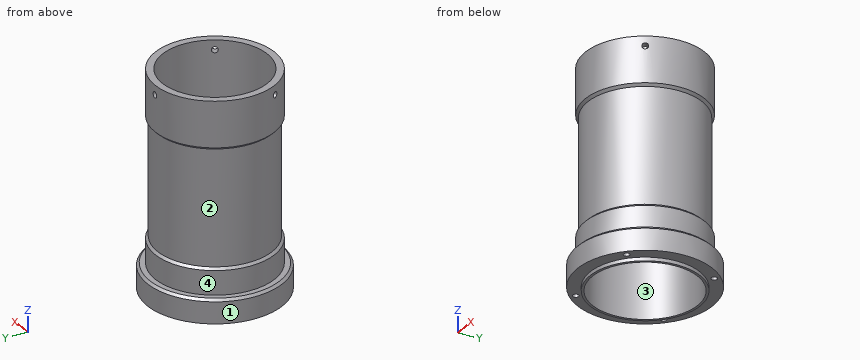
```python
from build123d import *

# Parameters (mm, degrees)
HOLE_WIZARD_M3_1_D       = 2.5
HOLE_WIZARD_M3_1_DEPTH   = 7
HOLE_WIZARD_M3_1_TIP     = 0.751075774
CHAMFER_2_SIZE           = 1
SKETCH_20_W              = 1.25
SKETCH_20_H              = 28.25
PATTERN_CIRCULAR_1_COUNT = 3


with BuildPart() as part:
    # 草图1 → 旋转1 (revolve)
    with BuildSketch(Plane(origin=(0, 0, 0), x_dir=(1, 0, 0), z_dir=(0, 1, 0))):
        Polygon((25, 0), (25, 19), (24, 19), (24, 69), (25, 69), (25, 79), (28.25, 79), (28.25, 89), (23, 89), (23, 90.5), (22, 90.5), (22, 0), align=None)
    revolve(axis=Axis((0, 0, 0), (0, 0, -1)))

    # M3 螺纹孔1
    with Locations(Plane(origin=(0, 0, -89), x_dir=(-1, 0, 0), z_dir=(0, 0, -1))):
        with Locations((-18.207999616, 18.207999616), (18.207999616, 18.207999616), (18.207999616, -18.207999616), (-18.207999616, -18.207999616)):
            Hole(HOLE_WIZARD_M3_1_D / 2, depth=HOLE_WIZARD_M3_1_DEPTH)
            with Locations((0, 0, -(HOLE_WIZARD_M3_1_DEPTH + HOLE_WIZARD_M3_1_TIP / 2))):  # 118° drill point
                Cone(0, HOLE_WIZARD_M3_1_D / 2, HOLE_WIZARD_M3_1_TIP, mode=Mode.SUBTRACT)

    # 倒角2
    chamfer_2_edges = [part.edges().sort_by_distance(p)[0] for p in [
        (-28.25, 0, -79),
        (-24, 0, -69),
        (-24, 0, -19),
    ]]
    chamfer(chamfer_2_edges, length=CHAMFER_2_SIZE - 0.0001)  # a hair under: the kernel refuses the full size

    # 草图20 → M3 螺纹孔2 (revolve, cut)
    with BuildSketch(Plane(origin=(0, 0, -4), x_dir=(0, 0, -1), z_dir=(1, 0, 0))):
        with Locations((0.625, 14.125)):
            Rectangle(SKETCH_20_W, SKETCH_20_H)
    hole_wizard_m3_2 = revolve(axis=Axis((0, -6.35, -4), (0, 1, 0)), mode=Mode.SUBTRACT)

    # 阵列(圆周)1: M3 螺纹孔2 ×3 about axis
    pattern_circular_1_axis = Axis((0, 0, 0), (0, 0, 1))
    for i in range(1, PATTERN_CIRCULAR_1_COUNT):
        add(hole_wizard_m3_2.rotate(pattern_circular_1_axis, i * 360 / PATTERN_CIRCULAR_1_COUNT), mode=Mode.SUBTRACT)


solid = part.part
```
Here's how the part is built. I have some questions about the finished solid (model axes, mm). Face numbers are marked on the shaded views. A direction names the side the tool comes from. Give positions to 0.01 mm unless a question says otherwise; leave off trailing zeros. Write each loop counter-clockwise with the first axis right and the second up, starting at its lowest first coordinate (ties: lowest second). Pieces come first, ordered by that corner, then holes.
(1) Thinking about a two-plate mould opening in Z: for the marked faces 1 and 2, which applies, pulls with the +Z half, pulls with the -Z half, needs draft (parallel to the pull), parting line crosses it, or undercut?
Output values:
face 1: needs draft
face 2: undercut
(2) Imagine slicing it at C-C, the plane z = -4. Write out the boundary of the cut face in (x, y), and give its area (3 significant figures).
Output values:
outline: (-22.25, -11.4) - (-19.65, -9.9) arc R22 cw to (-1.25, 21.96) - (-1.25, 24.97) arc R25 ccw to start; (-21, -13.57) arc R25 ccw to (21, -13.57) - (18.4, -12.06) arc R22 cw to (-18.4, -12.06) - close; (1.25, 21.96) arc R22 cw to (19.65, -9.9) - (22.25, -11.4) arc R25 ccw to (1.25, 24.97) - close
area: 420 mm2
(3) Imagine slicing it at B-B, the plane x = 0. Count the separate pieces of the cut face and the enclosed holes in it, and give its area (4 significant figures).
Output values:
separate pieces: 3
enclosed holes: 0
area: 495.5 mm2
(4) If I drill on L1, parallel to Y at x = 0, z = -18; L2, parallel to Y at x = -0.5, z = -60; L3, parallel to X at y = 0, z = -22, over which ranges is the centre line in solid material (lowest first)?
Output values:
L1: y = -25 to -22, 22 to 25
L2: y = -23.99 to -21.99, 21.99 to 23.99
L3: x = -24 to -22, 22 to 24
(5) Will these pins go through, and if not, where does the flat tip stop? pin 1 (10 mm diameter, centred on x = -21, z = -34.5, fed in from +Y); pin 2 (6 mm diameter, centred on x = -3, z = -46, fed in from +Y); pin 3 (3 mm diameter, centred on x = 18.208, y = -18.208, fed in from -Z).
Output values:
pin 1: stops at y = 17.89
pin 2: stops at y = 24
pin 3: stops at z = -89
(6) On a 3-axis mill with a long thin cutter (end or side, diameter ignored), from which of +Z, -Z, +X, -X, +Y, -Y can I reach the whole of each face in a straight line? I mean the marked faces 3 and 4. Say none if no direction works.
Output values:
face 3: +Z, -Z
face 4: +Z
